```python
from build123d import *

# Parameters (mm, degrees)
SKETCH_W        = 42.5
SKETCH_H        = 18.5
PAD_DEPTH       = 18.75
SKETCH001_W     = 40.5
SKETCH001_H     = 16.5
POCKET_DEPTH    = 18.75
POCKET001_DEPTH = 9.251
SKETCH003_W     = 34
SKETCH003_H     = 29
POCKET002_DEPTH = 0.1
POCKET003_DEPTH = 18.751
FILLET_R        = 5
FILLET001_R     = 1


with BuildPart() as part:
    # Sketch → Pad (new body, symmetric)
    with BuildSketch(Plane.XY):
        Rectangle(SKETCH_W, SKETCH_H)
    extrude(amount=PAD_DEPTH, both=True)

    # Sketch001 → Pocket (cut, symmetric)
    with BuildSketch(Plane.XY.offset(1)):
        Rectangle(SKETCH001_W, SKETCH001_H)
    extrude(amount=POCKET_DEPTH, both=True, mode=Mode.SUBTRACT)

    # Sketch002 → Pocket001 (cut, through all)
    with BuildSketch(Plane.XZ):
        with BuildLine():
            ThreePointArc((-12.5, 0), (0, -12.5), (12.5, 0))
            Line((12.5, 21.558593), (12.5, 0))
            Line((-12.5, 21.558593), (12.5, 21.558593))
            Line((-12.5, 0), (-12.5, 21.558593))
        make_face()
    extrude(amount=POCKET001_DEPTH, mode=Mode.SUBTRACT)

    # Sketch003 → Pocket002 (cut)
    with BuildSketch(Plane(origin=(0, 9.25, 0), x_dir=(-1, 0, 0), z_dir=(0, 1, 0))):
        Rectangle(SKETCH003_W, SKETCH003_H)
    extrude(amount=-POCKET002_DEPTH, mode=Mode.SUBTRACT)

    # Sketch004 → Pocket003 (cut, through all)
    with BuildSketch(Plane.XY):
        with BuildLine():
            ThreePointArc((-12.5, 6), (-18.5, 0), (-12.5, -6))
            Line((-12.5, -6), (12.5, -6))
            ThreePointArc((12.5, -6), (18.5, 0), (12.5, 6))
            Line((12.5, 6), (-12.5, 6))
        make_face()
    extrude(amount=-POCKET003_DEPTH, mode=Mode.SUBTRACT)

    # Fillet
    fillet_edges = [part.edges().sort_by_distance(p)[0] for p in [
        (-12.5, -8.75, 18.75),
        (12.5, -8.75, 18.75),
    ]]
    fillet(fillet_edges, radius=FILLET_R)

    # Fillet001
    fillet001_edges = [part.edges().sort_by_distance(p)[0] for p in [
        (-21.25, 9.25, 0),
        (-21.25, -9.25, 0),
        (21.25, -9.25, 0),
        (21.25, 9.25, 0),
        (-21.25, 0, -18.75),
        (0, -9.25, -18.75),
        (0, 9.25, -18.75),
        (21.25, 0, -18.75),
    ]]
    fillet(fillet001_edges, radius=FILLET001_R)


solid = part.part
```
CAD build for the part. Positions are in the model's coordinates, mm. A direction names the side the tool comes from. Round coordinates to 2 decimals unless told otherwise and drop trailing zeros. Order: outer loops, then holes, each group sorted by start corner. A loop starts at its lowest first (then second) coordinate and runs counter-clockwise, first axis right, second up.
Q1. Slice it at C-C (y = -5). Write the cut outline in (x, z).
Q2. Slice it at B-B (x = 0). Write the cut outline in (y, z).
Q3. Which spindle directions (+Z, -Z, +X, -X, +Y, -Y) get a long thin tool onto all of the face, cutting with end or side? Do faces 1 (the cylindrical face through (20.949, -8.965, 0.756)), 2 (the flat face through (-12.5, -9, 7)), 3 (the flat face through (0, 8.25, 1)), 4 (the cylindrical face through (-18.5, 0.1, -18.2)), 5 (the flat face through (0, 9.15, 0)). Say none if no direction does.
Q4. Two-plate mould, pull along X, no slides. Class faces 6 (the cylindrical face through (-20.965, 0.116, -18.449)), 7 (the flat face through (0, 6, -18)), 8 (the flat face through (1, -7, -18.75)): pulls with the +X half, pulls with the -X half, needs draft (parallel to the pull), parting line crosses it, or undercut.
Q5. Drop flat-ended pins along their axis: pin 1 (0.5 mm diameter, centred on x = -3.5, z = -18.5, fed in from +Y); pin 2 (2 mm diameter, centred on x = -10, y = -4, fed in from +Z); pin 3 (3 mm diameter, centred on x = 7.5, y = -7.5, fed in from +Z). Give the stop position or say it passes through.
Q6. Slice it at A-A (z = -15). Write the cut outline in (x, y), and give its area (3 significant figures).
Q7. Slice it at D-D (z = 2). Write the cut outline in (x, y), and give its area (3 significant figures).
Q8. Wall check: L1, parallel to X at y = 1, z = 5; L2, parallel to Y at x = -4, z = -15; L3, parallel to Y at x = 2, z = 16.5. Give the ranges that are in metal, low to high.
Results below:
1. outline: (-21.25, -17.75) arc R1 ccw to (-20.25, -18.75) - (-15.82, -18.75) - (-15.82, -17.75) - (-20.25, -17.75) - (-20.25, 18.75) - (-21.25, 18.75) - close; (15.82, -18.75) - (20.25, -18.75) arc R1 ccw to (21.25, -17.75) - (21.25, 18.75) - (20.25, 18.75) - (20.25, -17.75) - (15.82, -17.75) - close
2. outline: (-9.25, -17.75) arc R1 ccw to (-8.25, -18.75) - (-6, -18.75) - (-6, -17.75) - (-8.25, -17.75) - (-8.25, -12.5) - (-9.25, -12.5) - close; (6, -18.75) - (8.25, -18.75) arc R1 ccw to (9.25, -17.75) - (9.25, -14.5) - (9.15, -14.5) - (9.15, 14.5) - (9.25, 14.5) - (9.25, 18.75) - (8.25, 18.75) - (8.25, -17.75) - (6, -17.75) - close
3. face 1: +Z, -Z, +X, -Y
3. face 2: +Z, -Y
3. face 3: +Z
3. face 4: +Z, -Z
3. face 5: +Y
4. face 6: pulls with the -X half
4. face 7: undercut
4. face 8: needs draft
5. pin 1: stops at y = 9.12
5. pin 2: passes through
5. pin 3: stops at z = -8.88
6. outline: (-21.25, -8.25) arc R1 ccw to (-20.25, -9.25) - (20.25, -9.25) arc R1 ccw to (21.25, -8.25) - (21.25, 8.25) arc R1 ccw to (20.25, 9.25) - (-20.25, 9.25) arc R1 ccw to (-21.25, 8.25) - close; hole (-20.25, -8.25) - (20.25, -8.25) - (20.25, 8.25) - (-20.25, 8.25) - close
6. area: 117 mm2
7. outline: (-21.25, -8.25) arc R1 ccw to (-20.25, -9.25) - (-12.5, -9.25) - (-12.5, -8.25) - (-20.25, -8.25) - (-20.25, 8.25) - (20.25, 8.25) - (20.25, -8.25) - (12.5, -8.25) - (12.5, -9.25) - (20.25, -9.25) arc R1 ccw to (21.25, -8.25) - (21.25, 8.25) arc R1 ccw to (20.25, 9.25) - (17, 9.25) - (17, 9.15) - (-17, 9.15) - (-17, 9.25) - (-20.25, 9.25) arc R1 ccw to (-21.25, 8.25) - close
7. area: 88.7 mm2
8. L1: x = -21.25 to -20.25, 20.25 to 21.25
8. L2: y = -9.25 to -8.25, 8.25 to 9.25
8. L3: y = 8.25 to 9.25
